from build123d import *
from OCP.BRepFilletAPI import BRepFilletAPI_MakeChamfer

# Parameters (mm, degrees)
SKETCH1_W           = 44
SKETCH1_H           = 26
SKETCH1_R           = 1.6
BOSS_EXTRUDE1_DEPTH = 0.4
SKETCH2_W           = 44
SKETCH2_H           = 12
BOSS_EXTRUDE2_DEPTH = 0.4
CHAMFER1_SIZE       = 0.4
CHAMFER1_SIZE_2     = 0.335639852


with BuildPart() as part:
    # Sketch1 → Boss-Extrude1 (new body)
    with BuildSketch(Plane.XY):
        with Locations((22, 13)):
            Rectangle(SKETCH1_W, SKETCH1_H)
        with Locations((32, 3)):
            Circle(SKETCH1_R, mode=Mode.SUBTRACT)
        with Locations((12, 3)):
            Circle(SKETCH1_R, mode=Mode.SUBTRACT)
        with Locations((32, 23)):
            Circle(SKETCH1_R, mode=Mode.SUBTRACT)
        with Locations((12, 23)):
            Circle(SKETCH1_R, mode=Mode.SUBTRACT)
    extrude(amount=BOSS_EXTRUDE1_DEPTH)

    # Sketch2 → Boss-Extrude2 (add)
    with BuildSketch(Plane.XY.offset(0.4)):
        with Locations((22, 13)):
            Rectangle(SKETCH2_W, SKETCH2_H)
    extrude(amount=BOSS_EXTRUDE2_DEPTH)

    # Chamfer1
    chamfer1_edges_1 = [part.edges().sort_by_distance(p)[0] for p in [
        (22, 7, 0.4),
    ]]
    chamfer1_side_1 = [part.faces().sort_by_distance(p)[0] for p in [
        (22, 6.993287203, 0.4),
    ]]
    chamfer1_edges_2 = [part.edges().sort_by_distance(p)[0] for p in [
        (22, 19, 0.4),
    ]]
    chamfer1_side_2 = [part.faces().sort_by_distance(p)[0] for p in [
        (22, 19.006712797, 0.4),
    ]]
    chamfer1 = BRepFilletAPI_MakeChamfer(part.part.solid().wrapped)
    for e in chamfer1_edges_1:
        chamfer1.Add(CHAMFER1_SIZE - 0.0001, CHAMFER1_SIZE_2 - 0.0001, e.wrapped, chamfer1_side_1[0].wrapped)
    for e in chamfer1_edges_2:
        chamfer1.Add(CHAMFER1_SIZE_2 - 0.0001, CHAMFER1_SIZE - 0.0001, e.wrapped, chamfer1_side_2[0].wrapped)
    add(Compound.cast(chamfer1.Shape()), mode=Mode.REPLACE)  # a hair under: the kernel refuses the full size


solid = part.part
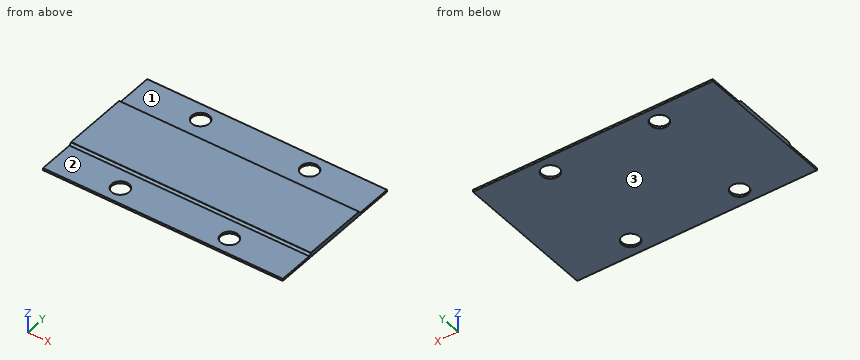
The model under review builds one solid part; all positions refer to its coordinate system, in mm. Face numbers are marked on the shaded views. A direction names the side the tool comes from. Give positions to 0.01 mm unless a question says otherwise; leave off trailing zeros. Loops run counter-clockwise (first coordinate to the right, second up) from the corner with the lowest first, then second, coordinate; pieces in that order, holes last. Notation, with made-up numbers: (6.5, 6) -> (39.5, 6) arc R21 ccw to (39.5, 13) -> close; hole circle Ø5 at (-9.5, 70.25). An arc over 180 degrees is marked (long way). Put each result on its own line as item: value. Start each with the question number.
1. Wall thickness on probe 1 along Y at (x, z) = (32, 0.15); probe 2 along X at (y, z) = (22.75, 0.35); probe 3 along Z at (x, y) = (19.5, 4.25): over which ranges is each line inside the solid? List them lowest first.
2. We need section C-C on x = 32. State how many separate pieces and enclosed holes the cut face has, then the cut area to 3 significant figures.
3. Clearance check with flat-ended pins moving along their axes: P1, Ø3.5, axis at x = 30, y = 22, coming from the +Z side; P2, Ø8, axis at x = 39, y = 19, coming from the -Z side. State where each tip first meets the part, or that it passes through.
4. We need section A-A on y = 23. State the section outline as (x, z) points, then the cut area to 3 significant figures.
5. For the marked faces 1, 2 and 3, list the 3-axis set-ups (+Z, -Z, +X, -X, +Y, -Y) from which the entire face can be reached by the end or side of a thin tool; tool diameter is ignored.
6. We need section B-B on z = 0.2. State the section outline as (x, y) points.
Determined:
1. probe 1: 0 to 1.4, 4.6 to 21.4, 24.6 to 26
1. probe 2: 0 to 10.42, 13.58 to 30.42, 33.58 to 44
1. probe 3: 0 to 0.4
2. separate pieces: 3
2. enclosed holes: 0
2. area: 12.8 mm^2
3. P1: z = 0.4
3. P2: z = 0
4. outline: (0, 0) -> (10.4, 0) -> (10.4, 0.4) -> (0, 0.4) -> close; (13.6, 0) -> (30.4, 0) -> (30.4, 0.4) -> (13.6, 0.4) -> close; (33.6, 0) -> (44, 0) -> (44, 0.4) -> (33.6, 0.4) -> close
4. area: 15.0 mm^2
5. face 1: +Z, +X, -X, +Y
5. face 2: +Z, +X, -X, -Y
5. face 3: -Z, +X, -X, +Y, -Y
6. outline: (0, 0) -> (44, 0) -> (44, 26) -> (0, 26) -> close; hole circle Ø3.2 at (12, 3); hole circle Ø3.2 at (12, 23); hole circle Ø3.2 at (32, 3); hole circle Ø3.2 at (32, 23)
